Here's how the part is built. I have some questions about the finished solid (model axes, mm). A direction names the side the tool comes from. Round coordinates to 2 decimals unless told otherwise and drop trailing zeros. Write each loop counter-clockwise with the first axis right and the second up, starting at its lowest first coordinate (ties: lowest second). Pieces come first, ordered by that corner, then holes. Notation, with made-up numbers: (3.25, 57) -> (8.25, 57) arc R17 cw to (8.25, 74) -> close; hole circle Ø10 at (-5.75, 66). An arc over 180 degrees is marked (long way). Answer as CSV lines item,"result".
from build123d import *

# Parameters (mm, degrees)
BASE_FLANGE1_DEPTH    = 10
FILLET1_R             = 3
SKETCH7_R             = 1.5
CUT_EXTRUDE1_DEPTH    = 39.171488051
BODY_MOVE_COPY1_ANGLE = 90


# Sheet-metal steps are written as plain solids
with BuildPart() as part:
    # Sketch1 → Base-Flange1 (new, symmetric)
    with BuildSketch(Plane.XY):
        with BuildLine():
            Line((-12, 0), (-2.75, 0))
            ThreePointArc((-2.75, 0), (-0.805456352, 0.805456352), (0, 2.75))
            Line((0, 2.75), (0, 15.5))
            ThreePointArc((0, 15.5), (0.219669914, 16.030330086), (0.75, 16.25))
            Line((0.75, 16.25), (32, 16.25))
            Line((32, 16.25), (32, 18.25))
            Line((32, 18.25), (0.75, 18.25))
            ThreePointArc((0.75, 18.25), (-1.194543648, 17.444543648), (-2, 15.5))
            Line((-2, 15.5), (-2, 2.75))
            ThreePointArc((-2, 2.75), (-2.219669914, 2.219669914), (-2.75, 2))
            Line((-2.75, 2), (-12, 2))
            Line((-12, 2), (-12, 0))
        make_face()
    extrude(amount=BASE_FLANGE1_DEPTH, both=True)

    # Fillet1
    fillet1_edges = [part.edges().sort_by_distance(p)[0] for p in [
        (32, 17.25, -10),
        (-12, 1, -10),
        (32, 17.25, 10),
        (-12, 1, 10),
    ]]
    fillet(fillet1_edges, radius=FILLET1_R)

    # Sketch7 → Cut-Extrude1 (cut, through all)
    with BuildSketch(Plane(origin=(0, 0, 0), x_dir=(1, 0, 0), z_dir=(0, 1, 0))):
        with BuildLine():
            Line((16.289213562, 0.5), (13.460786438, 0.5))
            ThreePointArc((13.460786438, 0.5), (14.621347032, -1.478397839), (16.375, 0))
            ThreePointArc((16.375, 0), (16.353397839, 0.253652968), (16.289213562, 0.5))
        make_face()
        with Locations((-9, -6)):
            Circle(SKETCH7_R)
        with Locations((-9, 6)):
            Circle(SKETCH7_R)
    extrude(amount=CUT_EXTRUDE1_DEPTH, mode=Mode.SUBTRACT)


with BuildPart() as part_1:
    # Body-Move/Copy1: moved
    add(part.part.rotate(Axis((0, 7.6, 0), (-1, 0, 0)), BODY_MOVE_COPY1_ANGLE))


solid = part_1.part
Item 1: For faces 1 (the flat face through (15, 7.1, -10)), 2 (the flat face through (-2, 8, -2)), 3 (the flat face through (7, 17.6, -9)), 4 (the flat face through (16, 6, -8.65)), which set-ups out of +Z, -Z, +X, -X, +Y, -Y let a thin tool reach every point of the face, with its end or its side?
Results found:
face 1,"+Z, -Z"
face 2,"-Z, -X, +Y, -Y"
face 3,"+Z, -Z, +X, -X, +Y"
face 4,"+Z, +X, +Y, -Y"
Item 2: Suppose I cut it at D-D, the plane y = 8.25. List the corners of the cut face in (x, z) for me, then the cut area to 3 significant figures.
Results found:
outline,"(-12, 5.6) -> (-2.75, 5.6) arc R0.75 cw to (-2, 4.85) -> (-2, -7.9) arc R2.75 ccw to (0.75, -10.65) -> (13.52, -10.65) -> (13.52, -8.65) -> (0.75, -8.65) arc R0.75 cw to (0, -7.9) -> (0, 4.85) arc R2.75 ccw to (-2.75, 7.6) -> (-12, 7.6) -> close; (16.23, -10.65) -> (32, -10.65) -> (32, -8.65) -> (16.23, -8.65) -> close"
area,"112 mm²"
Item 3: Suppose I cut it at C-C, the plane x = 6.5. List the corners of the cut face in (y, z) for me.
Results found:
outline,"(-2.4, -10.65) -> (17.6, -10.65) -> (17.6, -8.65) -> (-2.4, -8.65) -> close"
Item 4: If we mould it in two halves opening along X, with no side actions, what happens to faces 5 (the flat face through (7, -2.4, -9)), 6 (the cylindrical face through (31.14, -1.5, -9.66)), 7 (the cylindrical face through (-9.325, 15.064, 6.614))? For each: pulls with the +X half, pulls with the -X half, needs draft (parallel to the pull), parting line crosses it, or undercut.
Results found:
face 5,"needs draft"
face 6,"pulls with the +X half"
face 7,"undercut"
Item 5: Suppose I cut it at A-A, the plane y = 1.6. List the corners of the cut face in (x, z) for me.
Results found:
outline,"(-12, 5.6) -> (-10.5, 5.6) -> (-10.5, 7.6) -> (-12, 7.6) -> close; (-7.5, 5.6) -> (-2.75, 5.6) arc R0.75 cw to (-2, 4.85) -> (-2, -7.9) arc R2.75 ccw to (0.75, -10.65) -> (32, -10.65) -> (32, -8.65) -> (0.75, -8.65) arc R0.75 cw to (0, -7.9) -> (0, 4.85) arc R2.75 ccw to (-2.75, 7.6) -> (-7.5, 7.6) -> close"
Item 6: I need wall thicknesses on L1, parallel to Y at x = -9, z = 6.4; L2, parallel to X at y = 7.25, z = -7; L3, parallel to Z at x = 14, y = 2.75. Which ranges of each line are inside material? Lowest first, please.
Results found:
L1,"y = -2.4 to 0.1, 3.1 to 12.1, 15.1 to 17.6"
L2,"x = -2 to 0"
L3,"z = -10.65 to -8.65"
Item 7: Will these pins go through, and if not, where does the flat tip stop? pin 1 (6 mm diameter, centred on x = 24.5, y = 4, fed in from +Z); pin 2 (10 mm diameter, centred on y = 12, z = 5, fed in from +X); pin 3 (7.5 mm diameter, centred on x = -6.5, y = 4, fed in from -Z).
Results found:
pin 1,"stops at z = -8.65"
pin 2,"stops at x = 0"
pin 3,"stops at z = 5.6"
Item 8: Suppose I cut it at B-B, the plane y = 6. List the corners of the cut face in (x, z) for me.
Results found:
outline,"(-12, 5.6) -> (-2.75, 5.6) arc R0.75 cw to (-2, 4.85) -> (-2, -7.9) arc R2.75 ccw to (0.75, -10.65) -> (32, -10.65) -> (32, -8.65) -> (0.75, -8.65) arc R0.75 cw to (0, -7.9) -> (0, 4.85) arc R2.75 ccw to (-2.75, 7.6) -> (-12, 7.6) -> close"
